```python
from build123d import *

# Parameters (mm, degrees)
EXTRUDE_3_DEPTH = 46


with BuildPart() as part:
    # Эскиз3 → Бобышка-Вытянуть3 (new body)
    with BuildSketch(Plane.XY):
        with BuildLine():
            Line((11, 121.91), (11, 105.91))
            Line((11, 105.91), (36.91, 80))
            Line((36.91, 80), (131.533650814, 80))
            Line((131.533650814, 80), (153.572399359, 89.128748545))
            Line((153.572399359, 89.128748545), (164.886107858, 100.442457044))
            ThreePointArc((164.886107858, 100.442457044), (180.442457044, 100.442457044), (180.442457044, 84.886107858))
            Line((180.442457044, 84.886107858), (169.128748545, 73.572399359))
            Line((169.128748545, 73.572399359), (160, 51.533650814))
            Line((160, 51.533650814), (160, -51.533650814))
            Line((160, -51.533650814), (169.128748545, -73.572399359))
            Line((169.128748545, -73.572399359), (180.442457044, -84.886107858))
            ThreePointArc((180.442457044, -84.886107858), (180.442457044, -100.442457044), (164.886107858, -100.442457044))
            Line((164.886107858, -100.442457044), (153.572399359, -89.128748545))
            Line((153.572399359, -89.128748545), (131.533650814, -80))
            Line((131.533650814, -80), (36.91, -80))
            Line((36.91, -80), (11, -105.91))
            Line((11, -105.91), (11, -121.91))
            ThreePointArc((11, -121.91), (0, -132.91), (-11, -121.91))
            Line((-11, -121.91), (-11, -105.91))
            Line((-11, -105.91), (-36.91, -80))
            Line((-36.91, -80), (-131.533650814, -80))
            Line((-131.533650814, -80), (-153.572399359, -89.128748545))
            Line((-153.572399359, -89.128748545), (-164.886107858, -100.442457044))
            ThreePointArc((-164.886107858, -100.442457044), (-180.442457044, -100.442457044), (-180.442457044, -84.886107858))
            Line((-180.442457044, -84.886107858), (-169.128748545, -73.572399359))
            Line((-169.128748545, -73.572399359), (-160, -51.533650814))
            Line((-160, -51.533650814), (-160, 51.533650814))
            Line((-160, 51.533650814), (-169.128748545, 73.572399359))
            Line((-169.128748545, 73.572399359), (-180.442457044, 84.886107858))
            ThreePointArc((-180.442457044, 84.886107858), (-180.442457044, 100.442457044), (-164.886107858, 100.442457044))
            Line((-164.886107858, 100.442457044), (-153.572399359, 89.128748545))
            Line((-153.572399359, 89.128748545), (-131.533650814, 80))
            Line((-131.533650814, 80), (-36.91, 80))
            Line((-36.91, 80), (-11, 105.91))
            Line((-11, 105.91), (-11, 121.91))
            ThreePointArc((-11, 121.91), (0, 132.91), (11, 121.91))
        make_face()
    extrude(amount=EXTRUDE_3_DEPTH)


solid = part.part
```
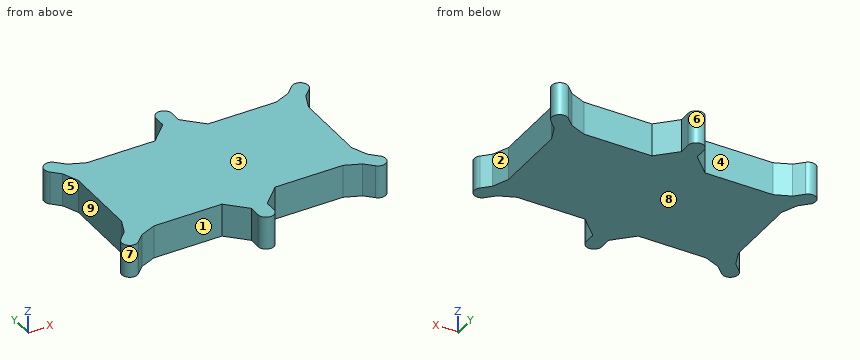
Build history of the part. All positions in model axes, mm. Face numbers are marked on the shaded views. A direction names the side the tool comes from. Give positions to 0.01 mm unless a question says otherwise; leave off trailing zeros. Loops run counter-clockwise (first coordinate to the right, second up) from the corner with the lowest first, then second, coordinate; pieces in that order, holes last. Notation, with made-up numbers: (64, -28.75) -> (68, -28.75) arc R23 cw to (68, -9.75) -> close; hole circle Ø6 at (23, 37.5). An arc over 180 degrees is marked (long way). One line per question, with ' | ' between items.
Q1. Cut at B-B, the plane x = 104. Write the cut outline in (y, z).
Filled sheet:
outline: (-80, 0) -> (80, 0) -> (80, 46) -> (-80, 46) -> close
Q2. Drop flat-ended pins along their axis: pin 1 (12 mm diameter, centred on y = -66.5, z = 26.5, fed in from -X); pin 2 (4 mm diameter, centred on x = 84.5, z = 11, fed in from +Y); pin 3 (8 mm diameter, centred on y = -117, z = 17, fed in from -X). Give the stop position or say it passes through.
Filled sheet:
pin 1: stops at x = -168.68 | pin 2: stops at y = 80 | pin 3: stops at x = -11
Q3. Drill centre lines: line 1 along X through (y, z) = (95, 16); line 2 along X through (y, z) = (90, 19.5); line 3 along X through (y, z) = (33, 14.5). Where is each one in solid material? Low to high. Write a range as [from, to].
Filled sheet:
line 1: x = [-183.41, -159.44], [-21.91, 21.91], [159.44, 183.41] | line 2: x = [-183.34, -154.44], [-26.91, 26.91], [154.44, 183.34] | line 3: x = [-160, 160]
Q4. Cut at A-A, the plane y = -28. Write the cut outline in (x, z).
Filled sheet:
outline: (-160, 0) -> (160, 0) -> (160, 46) -> (-160, 46) -> close
Q5. Pull direction X, two halves, no side cores. Call the marked faces 6, 7, 8 and 9: pulls with the +X half, pulls with the -X half, needs draft (parallel to the pull), parting line crosses it, or undercut.
Filled sheet:
face 6: parting line crosses it | face 7: undercut | face 8: needs draft | face 9: pulls with the -X half
Q6. Tool access for the marked faces 1, 2, 3, 4 and 5: list every direction of +Z, -Z, +X, -X, +Y, -Y with a clear straight run to the whole face (end or side of a thin tool).
Filled sheet:
face 1: +Z, -Z, -Y | face 2: +Z, -Z, +X | face 3: +Z, +X, -X, +Y, -Y | face 4: +Z, -Z, +Y | face 5: +Z, -Z, -X
